Autodesk Inventor part; units mm, degrees
ref_plane "YZ Plane" through (0, 0, 0) normal (1, 0, 0) x (0, 1, 0)
ref_plane "XZ Plane" through (0, 0, 0) normal (0, 1, 0) x (-1, 0, 0)
ref_plane "XY Plane" through (0, 0, 0) normal (0, 0, 1) x (1, 0, 0)
sketch "Sketch1" plane through (0, 0, 0) normal (0, 1, 0) x (-1, 0, 0)
  circle A0 centre (0, 0) radius 100
  dimension "d0" = 200
extrude "Extrusion1" add sketch "Sketch1" along normal blind 120
sketch "Sketch2" plane through (0, 0, 0) normal (0, -1, 0) x (1, 0, 0)
  line L0 (125, 125) -> (-125, 125)
  line L1 (-125, 125) -> (-125, -125)
  line L2 (-125, -125) -> (125, -125)
  line L3 (125, -125) -> (125, 125)
  line L4 (125, 125) -> (-125, -125) construction
  line L5 (-125, 125) -> (125, -125) construction
  point P0 (0, 0)
  dimension "d3" = 250
  dimension "d4" = 250
extrude "Extrusion2" add sketch "Sketch2" along normal blind 50
fillet "Fillet1" radius 20 1 edges at (100, 0, 0)
sketch "Sketch3" plane through (0, 120, 0) normal (0, 1, 0) x (1, 0, 0)
  circle A0 centre (0, 0) radius 87.5
  dimension "d8" = 175
extrude "Extrusion3" cut sketch "Sketch3" against normal blind 20
fillet "Fillet2" radius 10 1 edges at (-87.5, 120, 0)
sketch "Sketch4" plane through (0, 100, 0) normal (0, 1, 0) x (1, 0, 0)
  line L0 (-50, -50) -> (50, -50)
  line L1 (50, -50) -> (50, 50)
  line L2 (50, 50) -> (-50, 50)
  line L3 (-50, 50) -> (-50, -50)
  line L4 (-50, -50) -> (50, 50) construction
  line L5 (50, -50) -> (-50, 50) construction
  line L6 (-50, -50) -> (50, -50)
  line L7 (50, -50) -> (50, -20)
  line L8 (50, -20) -> (-50, -20)
  line L9 (-50, -20) -> (-50, -50)
  line L10 (-50, 50) -> (50, 50)
  line L11 (50, 50) -> (50, 20)
  line L12 (50, 20) -> (-50, 20)
  line L13 (-50, 20) -> (-50, 50)
  point P0 (0, 0)
  dimension "d12" = 100
  dimension "d13" = 100
  dimension "d14" = 30
  dimension "d15" = 30
extrude "Extrusion4" add sketch "Sketch4" along normal blind 125 contours L3 L8 L1 L0 | L3 L2 L1 L12
sketch "Sketch5" plane through (50, 100, -50) normal (0, 0, -1) x (-1, 0, 0)
  circle A0 centre (50, 75) radius 50
  line L0 (0, 0) -> (0, 125)
  line L1 (0, 75) -> (0, 125)
  line L2 (0, 125) -> (100, 125)
  line L3 (100, 125) -> (100, 75)
  circle A1 centre (50, 75) radius 25
  point P0 (50, -100)
  point P1 (50, 125)
  dimension "d18" = 50
extrude "Extrusion5" cut sketch "Sketch5" against normal blind 125 contours L0 L2 A0 | A0 L2 L3 | A1
fillet "Fillet3" radius 10 3 edges at (-50, 137.5, -20) (0, 225, -20) (50, 137.5, -20)
fillet "Fillet4" radius 10 3 edges at (0, 225, 20) (50, 137.5, 20) (-50, 137.5, 20)
fillet "Fillet5" radius 5 1 edges at (100, 120, 0)
fillet "Fillet6" radius 125 4 edges at (125, -25, 125) (125, -25, -125) (-125, -25, 125) (-125, -25, -125)
sketch "Sketch6" plane through (0, -50, 0) normal (0, -1, 0) x (1, 0, 0)
  circle A0 centre (0, 0) radius 60
  dimension "d25" = 120
extrude "Extrusion6" add sketch "Sketch6" along normal blind 10
properties part number "HANDBASE1"
Part model, mm, in its own coordinate system. A direction names the side the tool comes from. Give positions to 0.01 mm unless a question says otherwise; leave off trailing zeros. Write each loop counter-clockwise with the first axis right and the second up, starting at its lowest first coordinate (ties: lowest second). Pieces come first, ordered by that corner, then holes.
1) Cut at B-B on y = 190.5. State how many separate pieces and enclosed holes the cut face has, then the cut area to 3 significant figures.
Resolved:
separate pieces: 4
enclosed holes: 0
area: 3,260 mm2
2) Pin check, flat tips, straight feed: pin 1 (4 mm diameter, centred on x = -25, y = 59, fed in from +Z); pin 2 (4 mm diameter, centred on x = 82, y = 39, fed in from -Z); pin 3 (6 mm diameter, centred on y = 156, z = 38, fed in from +X). Stop position of each tip, or through.
Resolved:
pin 1: stops at z = 97.32
pin 2: stops at z = -60
pin 3: stops at x = 50
3) Cut at D-D on y = 72.5. Write the cut outline in (x, z).
Resolved:
outline: circle Ø200 at (0, 0)
4) Probe L1, parallel to Z at x = 0, y = 103; L2, parallel to Y at x = 0, z = 34; L3, parallel to Z at x = -16.5, y = 195. List the from-to ranges inside material, lowest first.
Resolved:
L1: z = -100 to -87.5, -50 to -20, 20 to 50, 87.5 to 100
L2: y = -60 to 150, 200 to 225
L3: z = -50 to -20, 20 to 50
5) Two-plate mould, pull along Y, no slides. Class faces 4 (the face through (-1, 148, 50)), 5 (the face through (3.255, 199.787, -35.21)), 6 (the face through (-1.099, 224.988, -40.14)): released by +Y, released by -Y, zero draft, split by the parting line, or undercut.
Resolved:
face 4: zero draft
face 5: undercut
face 6: released by +Y
6) Which spindle directions (+Z, -Z, +X, -X, +Y, -Y) get a long thin tool onto all of the face, cutting with end or side? Do faces 1 (the face through (-50, 137, 40)), 2 (the face through (-1, -60, 1)), 3 (the face through (-59.94, -54.93, -2.64)). Say none if no direction does.
Resolved:
face 1: +Y
face 2: +Z, -Z, +X, -X, -Y
face 3: -Y
